Can you work these out from the model? Positions are in its coordinate system, mm. Face numbers are marked on the shaded views. A direction names the side the tool comes from. Coordinates: 2 decimals unless noted, no trailing zeros. Loops run counter-clockwise (first coordinate to the right, second up) from the corner with the lowest first, then second, coordinate; pieces in that order, holes last. Notation, with made-up numbers: M 68,10 L 102,10 A15 cw 102,32 Z; hole C 72,61.25 d8. An arc over 180 degrees is marked long. Return JSON: item names as keys, results as strings. Group by question number.
```python
from build123d import *

# Parameters (mm, degrees)
SKETCH1_W           = 128.651
SKETCH1_H           = 67.2084
BOSS_EXTRUDE1_DEPTH = 42.6974
SKETCH2_W           = 115.951
SKETCH2_H           = 55.0164
CUT_EXTRUDE1_DEPTH  = 31.0134
SKETCH3_W           = 25.4
SKETCH3_H           = 4.684620624
CUT_EXTRUDE2_DEPTH  = 67.7164
SKETCH5_W           = 47.752
SKETCH5_H           = 23.185308257
CUT_EXTRUDE3_DEPTH  = 6.35


with BuildPart() as part:
    # Sketch1 → Boss-Extrude1 (new body)
    with BuildSketch(Plane(origin=(0, 0, 0), x_dir=(1, 0, 0), z_dir=(0, 1, 0))):
        with Locations((64.3255, 33.6042)):
            Rectangle(SKETCH1_W, SKETCH1_H)
    extrude(amount=BOSS_EXTRUDE1_DEPTH)

    # Sketch2 → Cut-Extrude1 (cut)
    with BuildSketch(Plane(origin=(0, 42.6974, 0), x_dir=(1, 0, 0), z_dir=(0, 1, 0))):
        with Locations((64.3255, 33.8582)):
            Rectangle(SKETCH2_W, SKETCH2_H)
    extrude(amount=-CUT_EXTRUDE1_DEPTH, mode=Mode.SUBTRACT)

    # Sketch3 → Cut-Extrude2 (cut)
    with BuildSketch(Plane.XY):
        with Locations((64.3255, 4.261689688)):
            Rectangle(SKETCH3_W, SKETCH3_H)
    extrude(amount=-CUT_EXTRUDE2_DEPTH, mode=Mode.SUBTRACT)

    # Sketch5 → Cut-Extrude3 (cut)
    with BuildSketch(Plane(origin=(128.651, 0, 0), x_dir=(0, 0, -1), z_dir=(1, 0, 0))):
        with Locations((32.004, 28.102654128)):
            Rectangle(SKETCH5_W, SKETCH5_H)
    cut_extrude3 = extrude(amount=-CUT_EXTRUDE3_DEPTH, mode=Mode.SUBTRACT)

    # Mirror1: Cut-Extrude3 across plane
    add(cut_extrude3.mirror(Plane.ZY.offset(-64.3255)), mode=Mode.SUBTRACT)


solid = part.part
```
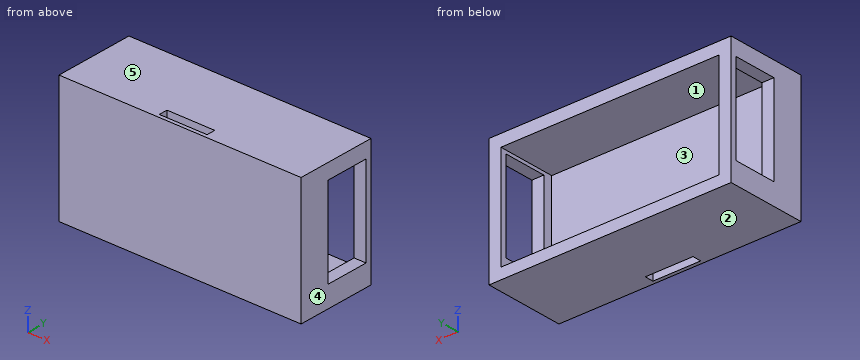
1) If we mould it in two halves opening along Z, with no side actions, what happens to the marked faces 3, 4 and 5? For each: +Z half, -Z half, draft (parallel to the pull), parting line (faces both ways), or undercut.
2) Suppose I cut it at D-D, the plane z = -5. List the corners of the cut face in (x, y) for me.
3) If I drill on line 1 (X direction, y = 30, z = -7.5); line 2 (Z direction, x = 6.5, y = 33), over which ranges is the centre line in solid material (lowest first)? Write a range as from..to.
4) For pin 1 (7.5 mm diameter, centred on x = 63.5, z = -49, fed in from +Y), with a flat end and sliding along its axis, tell me the tip position at first contact or that it passes through.
5) Suppose I cut it at B-B, the plane y = 4. List the corners of the cut face in (x, z) for me, then the cut area to 3 significant figures.
6) For the marked faces 1 and 2, which set-ups out of +Z, -Z, +X, -X, +Y, -Y let a thin tool reach every point of the face, with its end or its side?
7) Suppose I cut it at A-A, the plane z = -22. List the corners of the cut face in (x, y) for me, then the cut area to 3 significant figures.
8) Suppose I cut it at C-C, the plane x = 67.5. List the corners of the cut face in (y, z) for me, then the cut area to 3 significant figures.
Returned:
{
 "1": {"face 3": "undercut", "face 4": "draft", "face 5": "+Z half"},
 "2": {"outline": "M 0,0 L 128.65,0 L 128.65,42.7 L 0,42.7 Z; hole M 51.63,1.92 L 77.03,1.92 L 77.03,6.6 L 51.63,6.6 Z"},
 "3": {"line 1": "x = 0..6.35, 122.3..128.65", "line 2": "z = -67.21..-61.37, -6.35..0"},
 "4": {"pin 1": "stops at y = 11.68"},
 "5": {"outline": "M 0,-67.21 L 51.63,-67.21 L 51.63,0 L 0,0 Z; M 77.03,-67.21 L 128.65,-67.21 L 128.65,0 L 77.03,0 Z", "area": "6,940 mm²"},
 "6": {"face 1": "+Y", "face 2": "-Z, +X, -X, +Y, -Y"},
 "7": {"outline": "M 0,0 L 128.65,0 L 128.65,16.51 L 122.3,16.51 L 122.3,11.68 L 6.35,11.68 L 6.35,16.51 L 0,16.51 Z; M 0,39.7 L 6.35,39.7 L 6.35,42.7 L 0,42.7 Z; M 122.3,39.7 L 128.65,39.7 L 128.65,42.7 L 122.3,42.7 Z; hole M 51.63,1.92 L 77.03,1.92 L 77.03,6.6 L 51.63,6.6 Z", "area": "1,480 mm²"},
 "8": {"outline": "M 0,-67.21 L 1.92,-67.21 L 1.92,0 L 0,0 Z; M 6.6,-67.21 L 42.7,-67.21 L 42.7,-61.37 L 11.68,-61.37 L 11.68,-6.35 L 42.7,-6.35 L 42.7,0 L 6.6,0 Z", "area": "849 mm²"}
}
